CAD build for the part. Positions are in the model's coordinates, mm. A direction names the side the tool comes from. Round coordinates to 2 decimals unless told otherwise and drop trailing zeros. Loops run counter-clockwise (first coordinate to the right, second up) from the corner with the lowest first, then second, coordinate; pieces in that order, holes last. Notation, with made-up numbers: M -14.5,-24.5 L 8.5,-24.5 A20 ccw 8.5,-17.5 Z; hole C -9,7.25 d11. An arc over 180 degrees is marked long. Use a Markdown table: item, result. Add a question column.
(1) Flat gauge pins, fed straight in: P1, Ø4.5, axis at x = -1, z = 1, coming from the -Y side; P2, Ø2, axis at x = 3.5, y = 0.5, coming from the +Z side; P3, Ø0.5, axis at x = 0, z = 4, coming from the +Y side. Where does each tip first touch, or does it go through?
(2) Band-saw the part on C-C, the plane y = 0.65. Write the cut outline in (x, z).
(3) Band-saw the part on A-A, the plane x = 0. Write the cut outline in (y, z).
(4) Which spindle directions (+Z, -Z, +X, -X, +Y, -Y) get a long thin tool onto all of the face, cutting with end or side? Do faces 4 (the face through (0.02, -0.99, 4.31)), 5 (the face through (-0.078, 0.986, -5.562)), 6 (the face through (0, 1.9, -4)). Say none if no direction does.
(5) Wall check: L1, parallel to Y at x = -1.75, z = -4.25; L2, parallel to Y at x = -0.25, z = -4; L3, parallel to Z at x = -4, y = 0.6. Give the ranges that are in metal, low to high.
(6) Two-plate mould, pull along X, no slides. Class faces 1 (the face through (0, 1.9, 4)), 2 (the face through (-0.02, -0.99, -4.31)), 3 (the face through (0, 2, 0)): released by +X, released by -X, zero draft, split by the parting line, or undercut.
(7) Band-saw the part on B-B, the plane z = -3.81. Write the cut outline in (x, y).
(8) Band-saw the part on D-D, the plane z = 2. Write the cut outline in (x, y), and give its area (3 significant figures).
from build123d import *

# Parameters (mm, degrees)
BASE_EXTRUDE_DEPTH = 2
SKETCH2_R          = 0.5
PIN_EXTRUDE_DEPTH  = 2
SKETCH3_R          = 0.5
PIN_CUT_DEPTH      = 0.1


with BuildPart() as part:
    # Sketch1 → Base-Extrude (new body)
    with BuildSketch(Plane(origin=(0, 0, 0), x_dir=(1, 0, 0), z_dir=(0, 1, 0))):
        with BuildLine():
            Line((4.65, 3), (4.65, -3))
            ThreePointArc((4.65, -3), (0, -5.562739371), (-4.65, -3))
            Line((-4.65, -3), (-4.65, 3))
            ThreePointArc((-4.65, 3), (0, 5.562739371), (4.65, 3))
        make_face()
    extrude(amount=BASE_EXTRUDE_DEPTH)

    # Sketch2 → Pin-Extrude (add)
    with BuildSketch(Plane.XZ):
        with Locations(Location((0, 3.81, 0), (0, 0, 270))):
            Circle(SKETCH2_R)
        with Locations(Location((0, -3.81, 0), (0, 0, 90))):
            Circle(SKETCH2_R)
    extrude(amount=PIN_EXTRUDE_DEPTH)

    # Sketch3 → Pin-Cut (cut)
    with BuildSketch(Plane(origin=(0, 2, 0), x_dir=(1, 0, 0), z_dir=(0, 1, 0))):
        with Locations(Location((0, 3.81, 0), (0, 0, 270))):
            Circle(SKETCH3_R)
        with Locations(Location((0, -3.81, 0), (0, 0, 90))):
            Circle(SKETCH3_R)
    extrude(amount=-PIN_CUT_DEPTH, mode=Mode.SUBTRACT)


solid = part.part
Return value:
| question | item | result |
|---|---|---|
| 1 | P1 | y = 0 |
| 1 | P2 | z = 4.96 |
| 1 | P3 | y = 1.9 |
| 2 | outline | M -4.65,-3 A5.5 ccw 4.65,-3 L 4.65,3 A5.5 ccw -4.65,3 Z |
| 3 | outline | M -2,-4.31 L 0,-4.31 L 0,-5.56 L 2,-5.56 L 2,-4.31 L 1.9,-4.31 L 1.9,-3.31 L 2,-3.31 L 2,3.31 L 1.9,3.31 L 1.9,4.31 L 2,4.31 L 2,5.56 L 0,5.56 L 0,4.31 L -2,4.31 L -2,3.31 L 0,3.31 L 0,-3.31 L -2,-3.31 Z |
| 4 | face 4 | -Y |
| 4 | face 5 | -Z, +Y, -Y |
| 4 | face 6 | +Y |
| 5 | L1 | 0 to 2 |
| 5 | L2 | -2 to 1.9 |
| 5 | L3 | -3.84 to 3.84 |
| 6 | face 1 | undercut |
| 6 | face 2 | split by the parting line |
| 6 | face 3 | zero draft |
| 7 | outline | M -4.03,0 L -0.5,0 L -0.5,-2 L 0.5,-2 L 0.5,0 L 4.03,0 L 4.03,2 L 0.5,2 L 0.5,1.9 L -0.5,1.9 L -0.5,2 L -4.03,2 Z |
| 8 | outline | M -4.65,0 L 4.65,0 L 4.65,2 L -4.65,2 Z |
| 8 | area | 18.6 mm^2 |
